For this review, take the finished solid that the model builds, in its own axes (mm). A direction names the side the tool comes from. Round coordinates to 2 decimals unless told otherwise and drop trailing zeros. Loops run counter-clockwise (first coordinate to the right, second up) from the corner with the lowest first, then second, coordinate; pieces in that order, holes last.
1. To check wall thickness, follow line 1 along X through (y, z) = (-14.1, 15.5); line 2 along Z through (x, y) = (-11, -14.3); line 3 along Y through (x, z) = (29.3, 0) (3 decimals). State the ranges of each line that lie inside material, in increasing order.
2. Consider section D-D on x = -21.5. State the section outline as (y, z) points (3 decimals), then the cut area to 3 significant figures.
3. Consider section B-B on x = -11. State the section outline as (y, z) points, then the cut area to 3 significant figures.
4. Tool access review of faces 5 (the flat face through (29, 0, 0)), 6 (the flat face through (-24, 5.5, 0)), 7 (the flat face through (-25, 4, -4)), 8 (the flat face through (29, 4, -4)), 9 (the flat face through (-25, 4, 4)): name each direction out of +Z, -Z, +X, -X, +Y, -Y from which nothing blocks a thin tool from reaching the whole face with its end or side.
5. Consider section A-A on z = -15.5. State the section outline as (x, y) points, then the cut area to 3 significant figures.
6. Draft analysis for pull direction Y (two halves, no side actions). For faces 1 (the cylindrical face through (28.255, 1.126, -0.085)), 2 (the flat face through (30, 7, -3)), 3 (the flat face through (28, 8, 0)), 4 (the flat face through (28, 5.5, 0)), state which applies: released by +Y, released by -Y, zero draft, split by the parting line, or undercut.
7. Consider section C-C on x = -4. State the section outline as (y, z) points, then the cut area to 3 significant figures.
8. Clearance check with flat-ended pins moving along their axes: pin 1 Ø4.5 at (y, z) = (5, -2.5) entering from +X; pin 2 Ø2.5 at (x, z) = (-22.5, -1) entering from -Y; pin 3 Ø13 at (x, z) = (-5, -8) entering from +Y. State where each tip first meets the part, or that it passes through.
from build123d import *

# Parameters (mm, degrees)
SKETCH1_W                                           = 60
SKETCH1_H                                           = 8
BOSS_EXTRUDE1_DEPTH                                 = 8
BOSS_EXTRUDE2_DEPTH                                 = 17.5
BOSS_EXTRUDE2_DEPTH_BACK                            = 25.5
SKETCH5_W                                           = 43
SKETCH5_H                                           = 8
CUT_EXTRUDE2_DEPTH                                  = 17.5
SKETCH6_W                                           = 43
SKETCH6_H                                           = 8
BOSS_EXTRUDE3_DEPTH                                 = 2.5
SKETCH7_W                                           = 43
SKETCH7_H                                           = 8
BOSS_EXTRUDE4_DEPTH                                 = 2.5
CSK_FOR_M3_COUNTERSUNK_FLAT_HEAD_SCREW1_D           = 3.2
CSK_FOR_M3_COUNTERSUNK_FLAT_HEAD_SCREW1_CSINK_D     = 6.3
CSK_FOR_M3_COUNTERSUNK_FLAT_HEAD_SCREW1_CSINK_ANGLE = 90
SKETCH15_R                                          = 12.5
CUT_EXTRUDE3_DEPTH                                  = 5.5
CUT_EXTRUDE1_START                                  = -62.0000001
CUT_EXTRUDE1_DEPTH                                  = 62.0000001


with BuildPart() as part:
    # Sketch1 → Boss-Extrude1 (new body)
    with BuildSketch(Plane(origin=(0, 0, 0), x_dir=(1, 0, 0), z_dir=(0, 1, 0))):
        Rectangle(SKETCH1_W, SKETCH1_H)
    extrude(amount=BOSS_EXTRUDE1_DEPTH)

    # Sketch2 → Revolve1 (revolve)
    with BuildSketch(Plane(origin=(0, 4, 0), x_dir=(1, 0, 0), z_dir=(0, 1, 0))):
        with BuildLine():
            Line((30, 4), (30, 0))
            Line((30, 0), (31, 0))
            add(Edge.make_bspline(
                [(30, 4), (30.889676148, 2.05859871), (31, 0)],
                knots=[0, 0, 0, 1, 1, 1], degree=2))
        make_face()
    revolve1 = revolve(axis=Axis((30, 4, 0), (-1, 0, 0)))

    # Mirror1: Revolve1 across plane
    add(revolve1.mirror(Plane.ZY))

    # Sketch4 → Boss-Extrude2 (add, two sides: drawn at the far end of the back side and taken through both)
    with BuildSketch(Plane.XY.offset(4).offset(-BOSS_EXTRUDE2_DEPTH_BACK)):
        Polygon((28.5, 0), (26, 0), (26, -13.5), (-17, -13.5), (-17, 0), (-19.5, 0), (-19.5, -16.5), (28.5, -16.5), align=None)
    extrude(amount=BOSS_EXTRUDE2_DEPTH + BOSS_EXTRUDE2_DEPTH_BACK)

    # Sketch5 → Cut-Extrude2 (cut)
    with BuildSketch(Plane(origin=(0, 8, 0), x_dir=(1, 0, 0), z_dir=(0, 1, 0))):
        with Locations((4.5, 0)):
            Rectangle(SKETCH5_W, SKETCH5_H)
    extrude(amount=-CUT_EXTRUDE2_DEPTH, mode=Mode.SUBTRACT)

    # Sketch6 → Boss-Extrude3 (add)
    with BuildSketch(Plane.ZY.offset(-26)):
        with Locations((0, 4)):
            Rectangle(SKETCH6_W, SKETCH6_H)
    extrude(amount=-BOSS_EXTRUDE3_DEPTH)

    # Sketch7 → Boss-Extrude4 (add)
    with BuildSketch(Plane(origin=(-17, 0, 0), x_dir=(0, 0, -1), z_dir=(1, 0, 0))):
        with Locations((0, 4)):
            Rectangle(SKETCH7_W, SKETCH7_H)
    extrude(amount=-BOSS_EXTRUDE4_DEPTH)

    # CSK for M3 Countersunk Flat Head Screw1 (through all)
    with Locations(Plane(origin=(0, -16.5, 0), x_dir=(-1, 0, 0), z_dir=(0, -1, 0))):
        with Locations((11, -15.5), (-20, -15.5), (-20, 15.5), (11, 15.5)):
            CounterSinkHole(CSK_FOR_M3_COUNTERSUNK_FLAT_HEAD_SCREW1_D / 2, CSK_FOR_M3_COUNTERSUNK_FLAT_HEAD_SCREW1_CSINK_D / 2, counter_sink_angle=CSK_FOR_M3_COUNTERSUNK_FLAT_HEAD_SCREW1_CSINK_ANGLE)

    # Sketch15 → Cut-Extrude3 (cut)
    with BuildSketch(Plane(origin=(0, -16.5, 0), x_dir=(-1, 0, 0), z_dir=(0, -1, 0))):
        with Locations(Location((-4.5, 0, 0), (0, 0, 180))):
            Circle(SKETCH15_R)
    extrude(amount=-CUT_EXTRUDE3_DEPTH, mode=Mode.SUBTRACT)

    # Cut-Extrude1: read off the stored shape, not the designer's step
    # Cut-Extrude1 outline → Cut-Extrude1 (cut)
    with BuildSketch(Plane.ZY.offset(31).offset(CUT_EXTRUDE1_START)):
        with BuildLine():
            Line((2.452677109, 5.5), (-2.452677109, 5.5))
            ThreePointArc((-2.452677109, 5.5), (0, 1.125), (2.452677109, 5.5))
        make_face()
    extrude(amount=CUT_EXTRUDE1_DEPTH, mode=Mode.SUBTRACT)


solid = part.part
Resolved:
1. line 1: x = -19.5 to -12.6, -9.4 to 18.4, 21.6 to 28.5
1. line 2: z = -21.5 to -17.1, -13.9 to 13.9, 17.1 to 21.5
1. line 3: y = 0 to 1.125, 5.5 to 8
2. outline: (0, -4) - (8, -4) - (8, 4) - (0, 4) - close; hole (5.5, -2.453) - (5.5, 2.453) arc R2.875 ccw (long way) to start
2. area: 42.8 mm2
3. outline: (-16.5, -21.5) - (-13.5, -21.5) - (-13.5, -17.1) - (-14.95, -17.1) - (-16.5, -18.65) - close; (-16.5, -12.35) - (-14.95, -13.9) - (-13.5, -13.9) - (-13.5, 13.9) - (-14.95, 13.9) - (-16.5, 12.35) - close; (-16.5, 18.65) - (-14.95, 17.1) - (-13.5, 17.1) - (-13.5, 21.5) - (-16.5, 21.5) - close
3. area: 105 mm2
4. face 5: +Z, -Z, +X, -Y
4. face 6: +X, -X
4. face 7: -Z, -X, +Y, -Y
4. face 8: -Z, +X, +Y, -Y
4. face 9: +Z, -X, +Y, -Y
5. outline: (-19.5, -16.5) - (-14.15, -16.5) - (-12.6, -14.95) - (-12.6, -13.5) - (-17, -13.5) - (-17, 8) - (-19.5, 8) - close; (-9.4, -14.95) - (-7.85, -16.5) - (16.85, -16.5) - (18.4, -14.95) - (18.4, -13.5) - (-9.4, -13.5) - close; (21.6, -14.95) - (23.15, -16.5) - (28.5, -16.5) - (28.5, 8) - (26, 8) - (26, -13.5) - (21.6, -13.5) - close
5. area: 227 mm2
6. face 1: undercut
6. face 2: zero draft
6. face 3: released by +Y
6. face 4: undercut
7. outline: (-16.5, -21.5) - (-13.5, -21.5) - (-13.5, -9.17) - (-16.5, -9.17) - close; (-16.5, 9.17) - (-13.5, 9.17) - (-13.5, 21.5) - (-16.5, 21.5) - close
7. area: 74.0 mm2
8. pin 1: stops at x = 30.81
8. pin 2: stops at y = 0
8. pin 3: stops at y = -13.5
